Source: CAD feature listing. Evaluate the final solid. Frame: model axes, mm. A direction names the side the tool comes from. Give positions to 0.01 mm unless a question says otherwise; leave off trailing zeros. Order: outer loops, then holes, each group sorted by start corner. A loop starts at its lowest first (then second) coordinate and runs counter-clockwise, first axis right, second up.
```python
from build123d import *

# Parameters (mm, degrees)
SKETCH1_W           = 1500
SKETCH1_H           = 300
BOSS_EXTRUDE1_DEPTH = 50
SKETCH2_R           = 2.5
CUT_EXTRUDE1_DEPTH  = 50
SKETCH3_W           = 50
SKETCH3_H           = 200
CUT_EXTRUDE2_DEPTH  = 767.485485838


with BuildPart() as part:
    # Sketch1 → Boss-Extrude1 (new body)
    with BuildSketch(Plane(origin=(0, 0, 0), x_dir=(1, 0, 0), z_dir=(0, 1, 0))):
        Rectangle(SKETCH1_W, SKETCH1_H)
    extrude(amount=BOSS_EXTRUDE1_DEPTH)

    # Sketch2 → Cut-Extrude1 (cut)
    with BuildSketch(Plane.XY.offset(150)):
        with Locations((-650, 25)):
            Circle(SKETCH2_R)
        with Locations((-620, 25)):
            Circle(SKETCH2_R)
        with Locations((620, 25)):
            Circle(SKETCH2_R)
        with Locations((650, 25)):
            Circle(SKETCH2_R)
    extrude(amount=-CUT_EXTRUDE1_DEPTH, mode=Mode.SUBTRACT)

    # Sketch3 → Cut-Extrude2 (cut, through all)
    with BuildSketch(Plane(origin=(0, 50, 0), x_dir=(1, 0, 0), z_dir=(0, 1, 0))):
        with Locations((-525, 0)):
            Rectangle(SKETCH3_W, SKETCH3_H)
        with Locations((-325, 0)):
            Rectangle(SKETCH3_W, SKETCH3_H)
        with Locations((-125, 0)):
            Rectangle(SKETCH3_W, SKETCH3_H)
        with Locations((-25, 0)):
            Rectangle(SKETCH3_W, SKETCH3_H)
        with Locations((75, 0)):
            Rectangle(SKETCH3_W, SKETCH3_H)
        with Locations((175, 0)):
            Rectangle(SKETCH3_W, SKETCH3_H)
        with Locations((375, 0)):
            Rectangle(SKETCH3_W, SKETCH3_H)
        with Locations((575, 0)):
            Rectangle(SKETCH3_W, SKETCH3_H)
    extrude(amount=-CUT_EXTRUDE2_DEPTH, mode=Mode.SUBTRACT)


solid = part.part
```
1) Material intervals for L1, parallel to Y at x = 650, z = 127.5; L2, parallel to Z at x = -40, y = 16, sorted ascending.
Report:
L1: y = 0 to 22.5, 27.5 to 50
L2: z = -150 to -100, 100 to 150
2) Section query A-A, the plane x = 362.5. Return the cut outline in (y, z), and give its area (3 significant figures).
Report:
outline: (0, -150) - (50, -150) - (50, -100) - (0, -100) - close; (0, 100) - (50, 100) - (50, 150) - (0, 150) - close
area: 5,000 mm2
3) Reachability of faces 3 (the flat face through (575, 25, -100)), 4 (the flat face through (750, 25, 2)) from +Z, -Z, +X, -X, +Y, -Y: full face, straight path, thin tool, end or side. Return the list, or none.
Report:
face 3: +Y, -Y
face 4: +Z, -Z, +X, +Y, -Y
4) Pin query (flat end, axial travel): pin 1 (4 mm diameter, centred on x = 620.5, y = 24, fed in from +Z); pin 2 (1.5 mm diameter, centred on x = -619.5, y = 25.5, fed in from +Z). Return the tip coordinate at first contact, or that it passes through.
Report:
pin 1: stops at z = 150
pin 2: stops at z = 100
5) Draft query along Z for faces 1 (the flat face through (-125, 25, -100)), 2 (the flat face through (-10, 50, -102)). Return one class per face: +Z half, -Z half, draft (parallel to the pull), parting line (faces both ways), or undercut.
Report:
face 1: undercut
face 2: draft
6) Section query B-B, the plane y = 40. Count the separate pieces of the cut face and the enclosed holes in it, and give its area (3 significant figures).
Report:
separate pieces: 1
enclosed holes: 8
area: 370,000 mm2
